Read the model definition and answer for the solid it produces. Units are mm, in the model's axes. Coordinates: 2 decimals unless noted, no trailing zeros. Order: outer loops, then holes, each group sorted by start corner. A loop starts at its lowest first (then second) coordinate and runs counter-clockwise, first axis right, second up. Notation, with made-up numbers: M 86.5,-8 L 91.5,-8 A15 cw 91.5,-1 Z; hole C -12.5,32 d3. An arc over 180 degrees is marked long. Use a Markdown table: item, result. Add a question column.
1) Find section A-A on z = 9.5. Write down the section's boundary in (x, y), plus the area to 3 significant figures.
2) Find section C-C on x = -22. Write down the section's boundary in (y, z).
3) Find the intervals of material crossed by probe 1 along Z at (x, y) = (45, 0.8); probe 2 along Z at (x, y) = (-155, 0.9); probe 3 along X at (y, z) = (0.9, 37.5), in increasing order. Write a range as [from, to].
4) Find section D-D on x = 129. Write down the section's boundary in (y, z), plus the area to 3 significant figures.
5) Find section B-B on y = 1. Write down the section's boundary in (x, z).
6) Each of these flat-tipped pins is pushed along its axis until it touches: pin 1 Ø2.5 at (x, z) = (-155, 37.5) entering from +Y; pin 2 Ø0.8 at (x, y) = (-126.5, 0.5) entering from -Z. Where does it stop, or does it pass through?
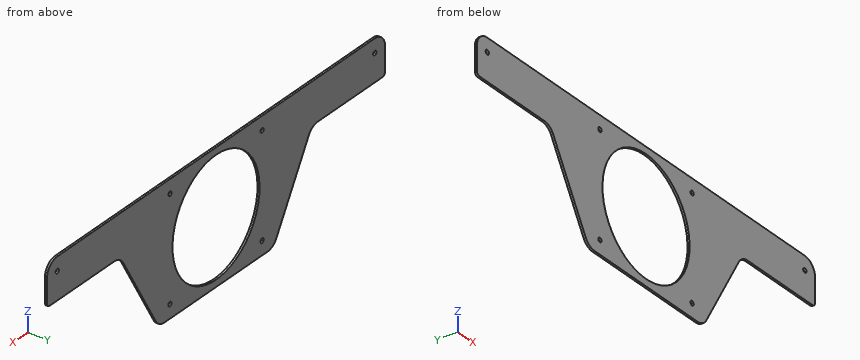
from build123d import *
from OCP.BRepFilletAPI import BRepFilletAPI_MakeFillet

# Parameters (mm, degrees)
ESQUISSE1_R             = 42.5
BOSS_EXTRU_1_DEPTH      = 1.5
CONG_1_R1               = 10
CONG_1_R2               = 2.5
ESQUISSE2_R             = 1.6
ENL_V_MAT_EXTRU_1_DEPTH = 172.707600298


with BuildPart() as part:
    # Esquisse1 → Boss.-Extru.1 (new body)
    with BuildSketch(Plane(origin=(0, 0, 0), x_dir=(1, 0, 0), z_dir=(0, 1, 0))):
        Polygon((56, 47.5), (-56, 47.5), (-93.527767497, -17.5), (-165, -17.5), (-165, -47.5), (165, -47.5), (165, -17.5), (93.527767497, -17.5), align=None)
        with Locations(Location((0, 0, 0), (0, 0, 270))):
            Circle(ESQUISSE1_R, mode=Mode.SUBTRACT)
    extrude(amount=BOSS_EXTRU_1_DEPTH)

    # Cong_1: one fillet with a radius per group of edges: ONE call of the kernel's fillet builder (fillet() takes one radius for all edges)
    cong_1_edges_1 = [part.edges().sort_by_distance(p)[0] for p in [
        (-165, 0.75, 47.5),
        (165, 0.75, 47.5),
        (-93.527767497, 0.75, 17.5),
        (-56, 0.75, -47.5),
        (56, 0.75, -47.5),
        (93.527767497, 0.75, 17.5),
    ]]
    cong_1_edges_2 = [part.edges().sort_by_distance(p)[0] for p in [
        (165, 0.75, 17.5),
        (-165, 0.75, 17.5),
    ]]
    cong_1 = BRepFilletAPI_MakeFillet(part.part.solid().wrapped)
    for e in cong_1_edges_1:
        cong_1.Add(CONG_1_R1, e.wrapped)
    for e in cong_1_edges_2:
        cong_1.Add(CONG_1_R2, e.wrapped)
    add(Compound.cast(cong_1.Shape()), mode=Mode.REPLACE)

    # Esquisse2 → Enl_v. mat.-Extru.1 (cut, through all)
    with BuildSketch(Plane(origin=(0, 1.5, 0), x_dir=(1, 0, 0), z_dir=(0, 1, 0))):
        with Locations(Location((-155, -37.5, 0), (0, 0, 270))):
            Circle(ESQUISSE2_R)
        with Locations(Location((-45, -37.5, 0), (0, 0, 270))):
            Circle(ESQUISSE2_R)
        with Locations(Location((-45, 37.5, 0), (0, 0, 270))):
            Circle(ESQUISSE2_R)
        with Locations(Location((45, -37.5, 0), (0, 0, 90))):
            Circle(ESQUISSE2_R)
        with Locations(Location((45, 37.5, 0), (0, 0, 90))):
            Circle(ESQUISSE2_R)
        with Locations(Location((155, -37.5, 0), (0, 0, 90))):
            Circle(ESQUISSE2_R)
    extrude(amount=-ENL_V_MAT_EXTRU_1_DEPTH, mode=Mode.SUBTRACT)


solid = part.part
Check result:
| question | item | result |
|---|---|---|
| 1 | outline | M -88.91,0 L -41.42,0 L -41.42,1.5 L -88.91,1.5 Z; M 41.42,0 L 88.91,0 L 88.91,1.5 L 41.42,1.5 Z |
| 1 | area | 142 mm2 |
| 2 | outline | M 0,-47.5 L 1.5,-47.5 L 1.5,-36.36 L 0,-36.36 Z; M 0,36.36 L 1.5,36.36 L 1.5,47.5 L 0,47.5 Z |
| 3 | probe 1 | z = [-47.5, -39.1], [-35.9, 35.9], [39.1, 47.5] |
| 3 | probe 2 | z = [17.5, 35.9], [39.1, 47.5] |
| 3 | probe 3 | x = [-165, -156.6], [-153.4, -46.6], [-43.4, -20], [20, 43.4], [46.6, 153.4], [156.6, 165] |
| 4 | outline | M 0,17.5 L 1.5,17.5 L 1.5,47.5 L 0,47.5 Z |
| 4 | area | 45.0 mm2 |
| 5 | outline | M -165,20 A2.5 ccw -162.5,17.5 L -99.3,17.5 A10 cw -90.64,12.5 L -58.89,-42.5 A10 ccw -50.23,-47.5 L 50.23,-47.5 A10 ccw 58.89,-42.5 L 90.64,12.5 A10 cw 99.3,17.5 L 162.5,17.5 A2.5 ccw 165,20 L 165,37.5 A10 ccw 155,47.5 L -155,47.5 A10 ccw -165,37.5 Z; hole C -155,37.5 d3.2; hole C -45,-37.5 d3.2; hole C -45,37.5 d3.2; hole C 0,0 d85; hole C 45,-37.5 d3.2; hole C 45,37.5 d3.2; hole C 155,37.5 d3.2 |
| 6 | pin 1 | passes through |
| 6 | pin 2 | stops at z = 17.5 |
